Input: part model. Units: mm. Frame: model coordinates. Face numbers are marked on the shaded views. A direction names the side the tool comes from. Round coordinates to 2 decimals unless told otherwise and drop trailing zeros. Loops run counter-clockwise (first coordinate to the right, second up) from the corner with the lowest first, then second, coordinate; pieces in that order, holes last. Notation, with made-up numbers: (17.25, -6) -> (61.25, -6) arc R20 ccw to (61.25, 25) -> close; hole circle Ø4 at (-8, 79). An arc over 180 degrees is marked (long way). Answer in a Markdown table with one row per item. Add a question column.
Q1. Reachability of the marked faces 1 and 2 from +Z, -Z, +X, -X, +Y, -Y: full face, straight path, thin tool, end or side. Return the list, or none.
Q2. Section B-B, the plane z = -2. Output: boundary loops of the cut face in (x, y), and give its area (3 significant figures).
Q3. Pin query (flat end, axial travel): pin 1 (5 mm diameter, centred on x = 11, y = 10.5, fed in from +Z); pin 2 (2 mm diameter, centred on x = 10, y = 14, fed in from -Z). Return the tip coordinate at first contact, or that it passes through.
Q4. Ray query, L1, parallel to Z at x = 9.5, y = 0; L2, parallel to Z at x = -19, y = 4.5; L3, parallel to X at y = -6, z = 1.5. Return the intervals inside material, ascending. Write a range as from..to.
Q5. Section A-A, the plane x = 0. Output: boundary loops of the cut face in (y, z).
```python
from build123d import *

# Parameters (mm, degrees)
SKETCH_1_R      = 25
EXTRUDE_1_DEPTH = 1
SKETCH_3_R      = 25
SKETCH_2_R      = 10
SKETCH_4_R      = 7.5
EXTRUDE_2_DEPTH = 1


with BuildPart() as part:
    # 草图1 → 凸台-拉伸1 (new body)
    with BuildSketch(Plane.XY):
        Circle(SKETCH_1_R)
    extrude(amount=EXTRUDE_1_DEPTH)

    # 草图3 → 放样1 section 0
    with BuildSketch(Plane(origin=(0, 0, 0), x_dir=(-1, 0, 0), z_dir=(0, 0, -1))):
        Circle(SKETCH_3_R)
    # 草图2 → 放样1 section 1
    with BuildSketch(Plane(origin=(0, 0, -5), x_dir=(-1, 0, 0), z_dir=(0, 0, -1))):
        Circle(SKETCH_2_R)
    loft()

    # 草图4 → 凸台-拉伸2 (add)
    with BuildSketch(Plane.XY.offset(1)):
        Circle(SKETCH_4_R)
    extrude(amount=EXTRUDE_2_DEPTH)


solid = part.part
```
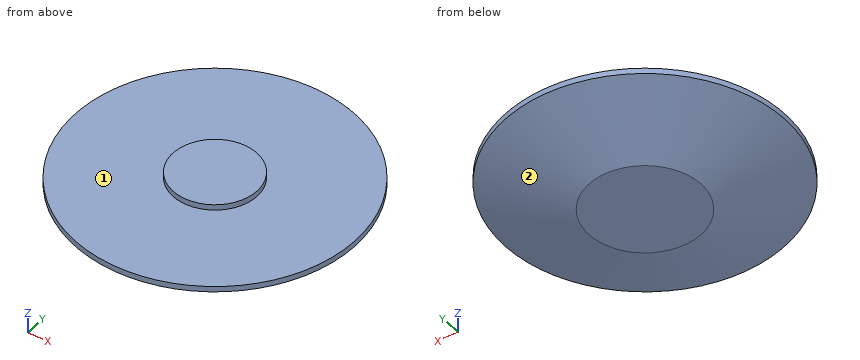
Answer block:
| question | item | result |
|---|---|---|
| 1 | face 1 | +Z |
| 1 | face 2 | -Z |
| 2 | outline | circle Ø38 at (0, 0) |
| 2 | area | 1,130 mm^2 |
| 3 | pin 1 | z = 1 |
| 3 | pin 2 | z = -2.93 |
| 4 | L1 | -5..1 |
| 4 | L2 | -1.82..1 |
| 4 | L3 | -4.5..4.5 |
| 5 | outline | (-25, 0) -> (-10, -5) -> (10, -5) -> (25, 0) -> (25, 1) -> (7.5, 1) -> (7.5, 2) -> (-7.5, 2) -> (-7.5, 1) -> (-25, 1) -> close |
